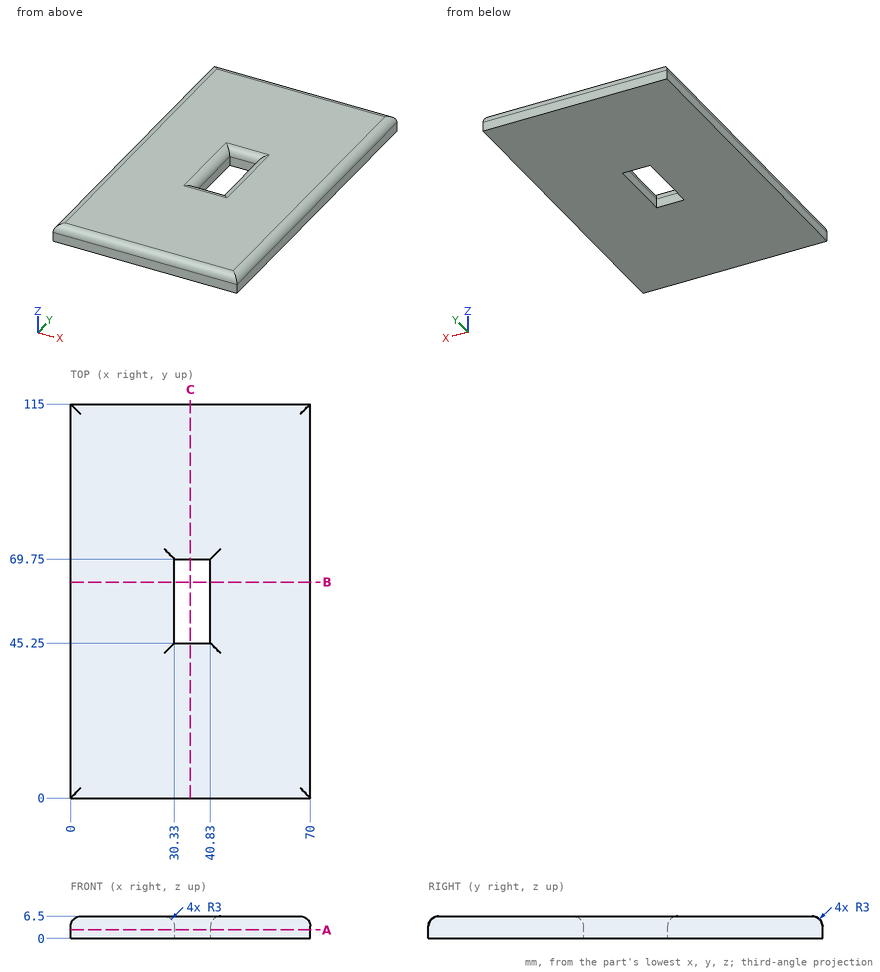
Print and shaded views of the part. All mm, measured from the part's lowest x, y and z. Round coordinates to 2 decimals unless told otherwise and drop trailing zeros. Order: outer loops, then holes, each group sorted by start corner. A loop starts at its lowest first (then second) coordinate and runs counter-clockwise, first axis right, second up.
Q1. Slice it at A-A (z = 2.5). Write the cut outline in (x, y).
Q2. Drop a flat-ended pin along its axis: pin 1 (1 mm diameter, centred on x = 49, z = 5, fed in from -Y). Give the stop position or say it passes through.
Q3. Slice it at C-C (x = 35). Write the cut outline in (y, z), and give its area (3 significant figures).
Q4. Wall check: L1, parallel to X at y = 55.5, z = 0.5; L2, parallel to Y at x = 33, z = 1.75; L3, parallel to X at y = 23.5, z = 5. Give the ranges that are in metal, low to high.
Q5. Slice it at B-B (y = 63). Write the cut outline in (x, z), and give its area (3 significant figures).
Results below:
1. outline: (0, 0) - (70, 0) - (70, 115) - (0, 115) - close; hole (30.33, 45.25) - (40.83, 45.25) - (40.83, 69.75) - (30.33, 69.75) - close
2. pin 1: stops at y = 0.17
3. outline: (0, 0) - (45.25, 0) - (45.25, 3.5) arc R3 ccw to (42.25, 6.5) - (3, 6.5) arc R3 ccw to (0, 3.5) - close; (69.75, 0) - (115, 0) - (115, 3.5) arc R3 ccw to (112, 6.5) - (72.75, 6.5) arc R3 ccw to (69.75, 3.5) - close
3. area: 581 mm2
4. L1: x = 0 to 30.33, 40.83 to 70
4. L2: y = 0 to 45.25, 69.75 to 115
4. L3: x = 0.4 to 69.6
5. outline: (0, 0) - (30.33, 0) - (30.33, 3.5) arc R3 ccw to (27.33, 6.5) - (3, 6.5) arc R3 ccw to (0, 3.5) - close; (40.83, 0) - (70, 0) - (70, 3.5) arc R3 ccw to (67, 6.5) - (43.83, 6.5) arc R3 ccw to (40.83, 3.5) - close
5. area: 379 mm2
